Input: part model. Units: mm. Frame: model coordinates. Give positions to 0.01 mm unless a question says otherwise; leave off trailing zeros. Answer as a JSON object with one key per item and string values. Group by question number.
1) First-contact query: P1, Ø5, axis at x = 4.5, z = -21, coming from the +Y side; P2, Ø4, axis at x = 2.5, y = -2.5, coming from the +Z side; P3, Ø1.5, axis at x = 4, z = -11.5, coming from the +Y side; P4, Ø2, axis at y = 5, z = 6, coming from the -X side. Flat tips, straight axial feed; report the tip coordinate or a pass-through.
2) Draft query along Z for faces 1 (the flat face through (0, 0, -25.325)), 2 (the conical face through (-4.996, 5.448, -23.359)), 3 (the flat face through (-6, -2, -15.566)). Return one class per face: +Z half, -Z half, draft (parallel to the pull), parting line (faces both ways), or undercut.
3) Ray query, L1, parallel to Z at x = -6.25, y = -4; L2, parallel to Z at x = 3.5, y = -5; L3, parallel to Z at x = 2.5, y = 2.75. Return the intervals inside material, ascending.
from build123d import *


with BuildPart() as f1:
    # F0 (on Right) → F1 (revolve)
    with BuildSketch(Plane.YZ):
        with BuildLine():
            Line((-6.743999, -15.566447), (-6.255512, -15.840568))
            ThreePointArc((-6.255512, -15.840568), (-8.376245, -19.305821), (-7.314796, -23.227405))
            Line((-7.314796, -23.227405), (-8.547529, -25.32473))
            Line((-8.547529, -25.32473), (0, -25.32473))
            Line((0, -25.32473), (0, 10.865145))
            ThreePointArc((0, 10.865145), (-0.859939, 10.400332), (-0.554096, 9.471889))
            ThreePointArc((-0.554096, 9.471889), (-3.106124, 4.850887), (-2.817132, -0.42007))
            ThreePointArc((-2.817132, -0.42007), (-3.149678, -0.799906), (-2.817132, -1.179742))
            Line((-2.817132, -1.179742), (-2.817132, -1.734666))
            Line((-2.817132, -1.734666), (-4.179219, -1.734666))
            Line((-4.179219, -1.734666), (-3.884023, -2.062576))
            ThreePointArc((-3.884023, -2.062576), (-4.44089, -2.78825), (-3.884023, -3.513924))
            ThreePointArc((-3.884023, -3.513924), (-4.089212, -9.668694), (-5.861165, -15.566447))
            Line((-5.861165, -15.566447), (-6.743999, -15.566447))
        make_face()
    revolve(axis=Axis((0, 0, -7.229792), (0, 0, -1)))


solid = f1.part
Output:
{
 "1": {"P1": "stops at y = 8.16", "P2": "stops at z = 8.32", "P3": "stops at y = 3.11", "P4": "passes through"},
 "2": {"face 1": "-Z half", "face 2": "undercut", "face 3": "+Z half"},
 "3": {"L1": "z = -25.32 to -23.41, -23.09 to -16.98", "L2": "z = -25.32 to -15.57", "L3": "z = -25.32 to -1.73"}
}
